For this review, use the dimensioned drawing (mm, ordinates from the lowest corner) and the shaded views. A direction names the side the tool comes from. Give positions to 0.01 mm unless a question says otherwise; leave off trailing zeros. Loops run counter-clockwise (first coordinate to the right, second up) from the corner with the lowest first, then second, coordinate; pieces in that order, holes last. Notation, with made-up numbers: (18, 34.25) -> (65, 34.25) arc R23 ccw to (65, 68.25) -> close; hole circle Ø7 at (-15, 54). An arc over 180 degrees is marked (long way). Write each question's results on one line, items separated by ' | '. Start each with the question number.
Q1. We need section D-D (x = 11.5). Write out the cut boundary in (y, z) (1 decimal).
Q2. Wall thickness on L1, parallel to X at y = 7.62, z = 11.7 (1 decimal); L2, parallel to X at y = 26, z = 10.5 (1 decimal); L3, parallel to X at y = 16.5, z = 6: over which ranges is each line inside the solid? List them lowest first. Write a range as [from, to].
Q3. We need section A-A (z = 11.5). Write out the cut boundary in (x, y) (1 decimal).
Q4. We need section B-B (y = 7.62). Write out the cut boundary in (x, z) (1 decimal).
Q5. We need section C-C (y = 21). Write out the cut boundary in (x, z).
Q6. Insertion check: pin 1 Ø0.8 at (x, z) = (2.5, 11) entering from +Y; pin 2 Ø3 at (y, z) = (23.5, 7) entering from -X; pin 3 Ø2 at (x, y) = (18, 22) entering from +Z; pin 4 Ø3 at (x, y) = (3.62, 7.62) entering from -Z. Each pin has a flat end and moves straight along its axis. Give the tip position at first contact, or say it passes through.
Q7. Mouldability with a two-part tool opening along X and no side actions: class the marked faces 5 and 6 as released by +X, released by -X, zero draft, split by the parting line, or undercut.
Q8. Machinability: for the marked faces 1, 2, 3 and 4, which of the approach directions +Z, -Z, +X, -X, +Y, -Y give a long, thin tool a straight path to every point of the face, cutting with its end or side? Answer none if there is none.
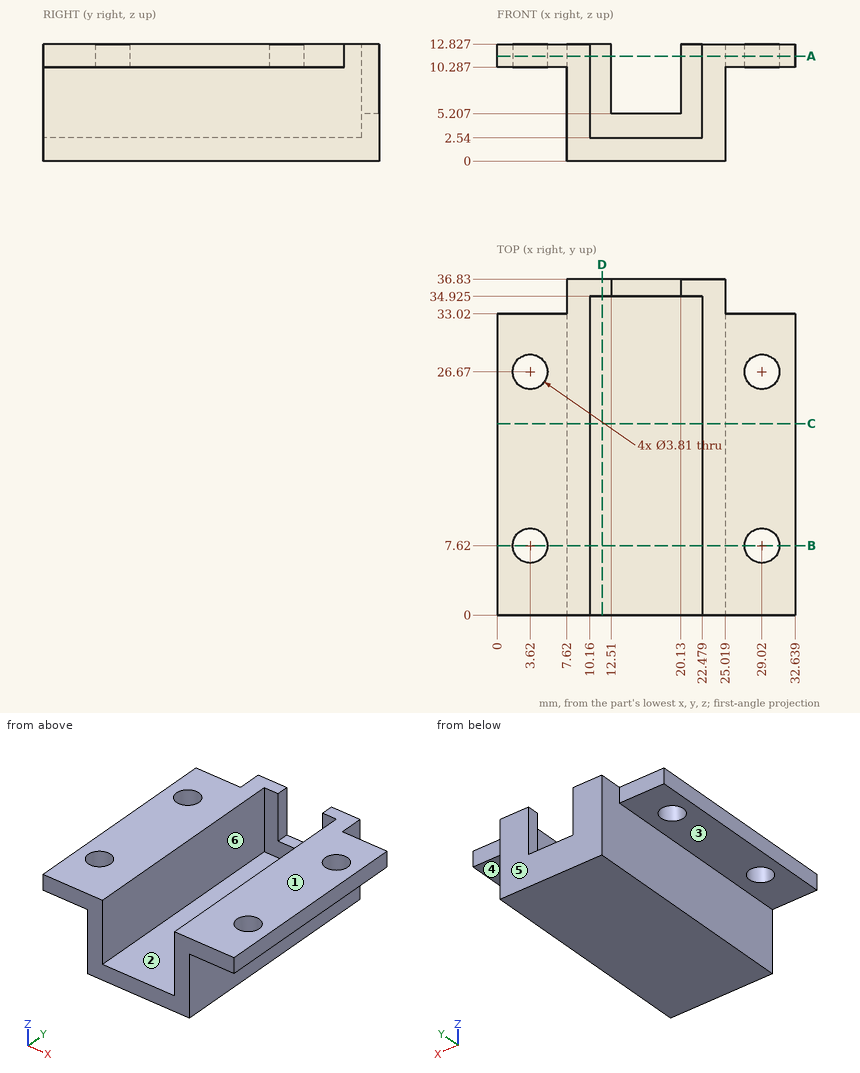
Output:
1) outline: (0, 0) -> (36.8, 0) -> (36.8, 12.8) -> (34.9, 12.8) -> (34.9, 2.5) -> (0, 2.5) -> close
2) L1: [0, 1.7], [5.5, 10.2], [22.5, 27.1], [30.9, 32.6] | L2: [0, 1.8], [5.4, 10.2], [22.5, 27.2], [30.8, 32.6] | L3: [7.62, 10.16], [22.48, 25.02]
3) outline: (0, 0) -> (10.2, 0) -> (10.2, 34.9) -> (12.5, 34.9) -> (12.5, 36.8) -> (7.6, 36.8) -> (7.6, 33) -> (0, 33) -> close; (20.1, 34.9) -> (22.5, 34.9) -> (22.5, 0) -> (32.6, 0) -> (32.6, 33) -> (25, 33) -> (25, 36.8) -> (20.1, 36.8) -> close; hole circle Ø3.8 at (3.6, 7.6); hole circle Ø3.8 at (3.6, 26.7); hole circle Ø3.8 at (29, 7.6); hole circle Ø3.8 at (29, 26.7)
4) outline: (0, 10.3) -> (1.7, 10.3) -> (1.7, 12.8) -> (0, 12.8) -> close; (5.5, 10.3) -> (7.6, 10.3) -> (7.6, 0) -> (25, 0) -> (25, 10.3) -> (27.1, 10.3) -> (27.1, 12.8) -> (22.5, 12.8) -> (22.5, 2.5) -> (10.2, 2.5) -> (10.2, 12.8) -> (5.5, 12.8) -> close; (30.9, 10.3) -> (32.6, 10.3) -> (32.6, 12.8) -> (30.9, 12.8) -> close
5) outline: (0, 10.29) -> (7.62, 10.29) -> (7.62, 0) -> (25.02, 0) -> (25.02, 10.29) -> (32.64, 10.29) -> (32.64, 12.83) -> (22.48, 12.83) -> (22.48, 2.54) -> (10.16, 2.54) -> (10.16, 12.83) -> (0, 12.83) -> close
6) pin 1: y = 33.02 | pin 2: x = 7.62 | pin 3: z = 2.54 | pin 4: through
7) face 5: zero draft | face 6: undercut
8) face 1: +Z, +X, -X, +Y, -Y | face 2: +Z, -Y | face 3: -Z, -X, +Y, -Y | face 4: -Z, +X, +Y, -Y
